```python
from build123d import *

# Parameters (mm, degrees)
F0_R     = 3.25
F0_W     = 31.5
F0_H     = 13
F0_W_2   = 51
F1_DEPTH = 2
F2_DEPTH = 2


# Not quite as in the source:
# - a feature names something its author has since deleted; it is built from what else it names


with BuildPart() as f1:
    # F0 (on Top) → F1 (new body)
    with BuildSketch(Plane.XY):
        Polygon((-26.2163661122, 15.2858447556), (-43.2163661122, 15.2858447556), (-43.2163661122, -26.4641552444), (-26.2163661122, -26.4641552444), (-26.2163661122, -11.9641552444), (-26.2163661122, 1.0358447556), align=None)
        with Locations((-35.2163661122, -19.2141552444)):
            Circle(F0_R, mode=Mode.SUBTRACT)
        with Locations((-35.2163661122, 0.7858447556)):
            Circle(F0_R, mode=Mode.SUBTRACT)
        Polygon((22.2836338878, 15.2858447556), (5.2836338878, 15.2858447556), (5.2836338878, 1.0358447556), (5.2836338878, -11.9641552444), (5.2836338878, -26.4641552444), (22.2836338878, -26.4641552444), (22.2836338878, -12.2141552444), (22.2836338878, 0.7858447556), align=None)
        with Locations((13.7836338878, -19.2141552444)):
            Circle(F0_R, mode=Mode.SUBTRACT)
        with Locations((13.7836338878, 0.7858447556)):
            Circle(F0_R, mode=Mode.SUBTRACT)
        Polygon((90.2836338878, -26.4641552444), (90.2836338878, 15.2858447556), (73.2836338878, 15.2858447556), (73.2836338878, 0.7858447556), (73.2836338878, -12.2141552444), (73.2836338878, -26.4641552444), align=None)
        with Locations((81.7836338878, -19.2141552444)):
            Circle(F0_R, mode=Mode.SUBTRACT)
        with Locations((81.7836338878, 0.7858447556)):
            Circle(F0_R, mode=Mode.SUBTRACT)
        Polygon((-26.2163661122, -26.4641552444), (-43.2163661122, -26.4641552444), (-43.2163661122, -36.4641552444), (90.2836338878, -36.4641552444), (90.2836338878, -26.4641552444), (73.2836338878, -26.4641552444), (22.2836338878, -26.4641552444), (5.2836338878, -26.4641552444), align=None)
        with Locations((-10.4663661122, -5.4641552444)):
            Rectangle(F0_W, F0_H)
        with Locations((47.7836338878, -5.7141552444)):
            Rectangle(F0_W_2, F0_H)
    extrude(amount=F1_DEPTH)

    # F0 (on Top) → F2 (join)
    with BuildSketch(Plane.XY):
        Polygon((90.2836338878, 28.2858447556), (-43.2163661122, 28.2858447556), (-43.2163661122, 15.2858447556), (-26.2163661122, 15.2858447556), (5.2836338878, 15.2858447556), (22.2836338878, 15.2858447556), (73.2836338878, 15.2858447556), (90.2836338878, 15.2858447556), align=None)
        with Locations((-35.2163661122, 21.7858447556)):
            Circle(F0_R, mode=Mode.SUBTRACT)
        with Locations((13.7836338878, 21.7858447556)):
            Circle(F0_R, mode=Mode.SUBTRACT)
        with Locations((81.7836338878, 21.7858447556)):
            Circle(F0_R, mode=Mode.SUBTRACT)
    extrude(amount=F2_DEPTH)


solid = f1.part
```
Here's how the part is built. I have some questions about the finished solid (model axes, mm). Coordinates: 2 decimals unless noted, no trailing zeros. Loops run counter-clockwise (first coordinate to the right, second up) from the corner with the lowest first, then second, coordinate; pieces in that order, holes last. Notation, with made-up numbers: (73, 72) -> (101, 72) arc R23 ccw to (101, 104) -> close; hole circle Ø11 at (36.5, -38.75). An arc over 180 degrees is marked (long way). Return JSON: item names as keys, results as strings.
1) If we section it at D-D, the plane z = 1.35: Count the separate pieces of the cut face and the enclosed holes in it, then the cut area to 3 significant figures.
Results below:
{"separate pieces": "1", "enclosed holes": "13", "area": "5,970 mm²"}
2) If we section it at B-B, the plane y = 7: Write out the boundary of the cut face in (x, z).
Results below:
{"outline": "(-43.22, 0) -> (-26.22, 0) -> (-26.22, 2) -> (-43.22, 2) -> close; (5.28, 0) -> (22.28, 0) -> (22.28, 2) -> (5.28, 2) -> close; (73.28, 0) -> (90.28, 0) -> (90.28, 2) -> (73.28, 2) -> close"}
3) Thinking about a two-plate mould opening in X: for faces 1 (the face through (23, -4, 0)), 2 (the face through (78.537, -19.071, 0.986)), 3 (the face through (-33.469, -16.474, 0.986)), which applies, +X half, -X half, draft (parallel to the pull), parting line (faces both ways), or undercut?
Results below:
{"face 1": "draft", "face 2": "undercut", "face 3": "undercut"}
4) I need wall thicknesses on line 1 (Y direction, x = 31, z = 1.3); line 2 (X direction, y = -14, z = 1.6); line 3 (Y direction, x = -15, z = 0.8). Which ranges of each line are inside material? Lowest first, please. Write a range as from..to.
Results below:
{"line 1": "-36.46..-26.46, -12.21..0.79, 15.29..28.29", "line 2": "-43.22..-26.22, 5.28..22.28, 73.28..90.28", "line 3": "-36.46..-26.46, -11.96..1.04, 15.29..28.29"}
5) If we section it at C-C, the plane y = -1: Write out the boundary of the cut face in (x, z), then the cut area to 3 significant figures.
Results below:
{"outline": "(-43.22, 0) -> (-37.93, 0) -> (-37.93, 2) -> (-43.22, 2) -> close; (-32.5, 0) -> (11.07, 0) -> (11.07, 2) -> (-32.5, 2) -> close; (16.5, 0) -> (79.07, 0) -> (79.07, 2) -> (16.5, 2) -> close; (84.5, 0) -> (90.28, 0) -> (90.28, 2) -> (84.5, 2) -> close", "area": "234 mm²"}
6) If we section it at A-A, the plane x = 24.5: Write out the boundary of the cut face in (y, z), then the cut area to 3 significant figures.
Results below:
{"outline": "(-36.46, 0) -> (-26.46, 0) -> (-26.46, 2) -> (-36.46, 2) -> close; (-12.21, 0) -> (0.79, 0) -> (0.79, 2) -> (-12.21, 2) -> close; (15.29, 0) -> (28.29, 0) -> (28.29, 2) -> (15.29, 2) -> close", "area": "72.0 mm²"}
